Read the model definition and answer for the solid it produces. Units are mm, in the model's axes. Face numbers are marked on the shaded views. A direction names the side the tool comes from. Coordinates: 2 decimals unless noted, no trailing zeros. Loops run counter-clockwise (first coordinate to the right, second up) from the corner with the lowest first, then second, coordinate; pieces in that order, holes last. Notation, with made-up numbers: (-11.75, 72) -> (13.25, 72) arc R23 ccw to (13.25, 99) -> close; hole circle Ø10 at (62.25, 24). An arc over 180 degrees is marked (long way). Answer as a JSON object with one key per item and string values. Group by question number.
Q1. The part is cut by section C-C on y = 10. Write down the section's boundary in (x, z).
Q2. Determine the mould class of the marked faces 1, 2 and 3 for opening direction X: released by +X, released by -X, zero draft, split by the parting line, or undercut.
Q3. Each of these flat-tipped pins is pushed along its axis until it touches: P1, Ø1.2, axis at x = 0.5, y = 19, coming from the +Z side; P2, Ø2, axis at x = 5, z = 9, coming from the +Y side; P3, Ø2, axis at x = 2.5, z = 9.5, coming from the -Y side; P4, Ø4, axis at x = 5, z = 9.5, coming from the -Y side. Where does it stop, or does it pass through?
Q4. The part is cut by section B-B on x = 0. Write down the section's boundary in (y, z).
Q5. Straight lines are drawn through the part: line 1 along Z through (x, y) = (7, 15.75); line 2 along X through (y, z) = (4.25, 5); line 3 along Y through (x, z) = (-9, 6.75). For each, find the intervals that lie inside material, in ascending order. Write a range as [from, to].
Q6. For the marked faces 4, 5, 6 and 7, determine the directions among +Z, -Z, +X, -X, +Y, -Y from which every point of the face is accessible in a straight line to the end or side of a thin tool.
from build123d import *

# Parameters (mm, degrees)
CYLINDER003_R     = 1.5
CYLINDER003_DEPTH = 40
ARRAY001_COUNT    = 8
CYLINDER002_R     = 10
CYLINDER002_DEPTH = 15
CHAMFER_SIZE      = 1
CHAMFER001_SIZE   = 1
CHAMFER002_SIZE   = 1
CHAMFER003_SIZE   = 1
CHAMFER004_SIZE   = 1
CHAMFER005_SIZE   = 1
CHAMFER006_SIZE   = 1
CHAMFER007_SIZE   = 1


with BuildPart() as array001:
    # Cylinder003 → Cylinder003 (new body)
    with BuildSketch(Plane.XY):
        Circle(CYLINDER003_R)
    extrude(amount=CYLINDER003_DEPTH)

    # Array001: Array001 ×8 about axis
    array001_axis = Axis((0, 10, 0), (0, 0, 1))


with BuildPart() as array001_1:
    add(array001.part)
    for i in range(1, ARRAY001_COUNT):
        add(array001.part.rotate(array001_axis, i * 360 / ARRAY001_COUNT))


with BuildPart() as array001_2:
    # Array001 placement: moved
    add(array001_1.part.moved(Location((0, 0, 3))))


with BuildPart() as chamfer007:
    # Cylinder002 → Cylinder002 (new body)
    with BuildSketch(Plane(origin=(0, 10, 0), x_dir=(1, 0, 0), z_dir=(0, 0, 1))):
        Circle(CYLINDER002_R)
    extrude(amount=CYLINDER002_DEPTH)

    # Cut001: cut Array001
    add(array001_2.part, mode=Mode.SUBTRACT)

    # Chamfer
    chamfer_edges = [chamfer007.edges().sort_by_distance(p)[0] for p in [
        (-3.826834, 0.761205, 15),
    ]]
    chamfer(chamfer_edges, length=CHAMFER_SIZE)

    # Chamfer001
    chamfer001_edges = [chamfer007.edges().sort_by_distance(p)[0] for p in [
        (3.826834, 0.761205, 15),
    ]]
    chamfer(chamfer001_edges, length=CHAMFER001_SIZE)

    # Chamfer002
    chamfer002_edges = [chamfer007.edges().sort_by_distance(p)[0] for p in [
        (-9.238795, 6.173166, 15),
    ]]
    chamfer(chamfer002_edges, length=CHAMFER002_SIZE)

    # Chamfer003
    chamfer003_edges = [chamfer007.edges().sort_by_distance(p)[0] for p in [
        (9.238795, 6.173166, 15),
    ]]
    chamfer(chamfer003_edges, length=CHAMFER003_SIZE)

    # Chamfer004
    chamfer004_edges = [chamfer007.edges().sort_by_distance(p)[0] for p in [
        (9.238795, 13.826834, 15),
    ]]
    chamfer(chamfer004_edges, length=CHAMFER004_SIZE)

    # Chamfer005
    chamfer005_edges = [chamfer007.edges().sort_by_distance(p)[0] for p in [
        (3.826834, 19.238795, 15),
    ]]
    chamfer(chamfer005_edges, length=CHAMFER005_SIZE)

    # Chamfer006
    chamfer006_edges = [chamfer007.edges().sort_by_distance(p)[0] for p in [
        (-9.238795, 13.826834, 15),
    ]]
    chamfer(chamfer006_edges, length=CHAMFER006_SIZE)

    # Chamfer007
    chamfer007_edges = [chamfer007.edges().sort_by_distance(p)[0] for p in [
        (-3.826834, 19.238795, 15),
    ]]
    chamfer(chamfer007_edges, length=CHAMFER007_SIZE)


solid = chamfer007.part
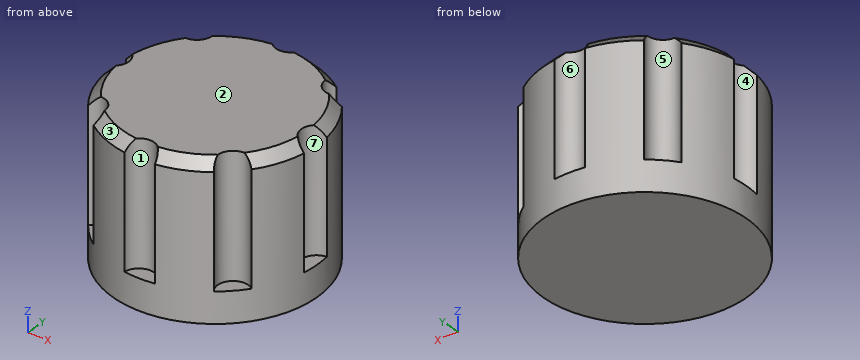
Final values:
{
 "1": {"outline": "(-10, 0) -> (10, 0) -> (10, 3) -> (8.5, 3) -> (8.5, 15) -> (-8.5, 15) -> (-8.5, 3) -> (-10, 3) -> close"},
 "2": {"face 1": "undercut", "face 2": "zero draft", "face 3": "released by -X"},
 "3": {"P1": "stops at z = 15", "P2": "stops at y = 19.17", "P3": "stops at y = 0.11", "P4": "stops at y = 0.46"},
 "4": {"outline": "(0, 0) -> (20, 0) -> (20, 3) -> (18.5, 3) -> (18.5, 15) -> (1.5, 15) -> (1.5, 3) -> (0, 3) -> close"},
 "5": {"line 1": "z = [0, 3]", "line 2": "x = [-8.18, -7.78], [-6.36, 6.36], [7.78, 8.18]", "line 3": "y = [5.64, 8.88], [11.12, 14.36]"},
 "6": {"face 4": "+Z, -X", "face 5": "+Z", "face 6": "+Z, +Y", "face 7": "+Z, +X"}
}
